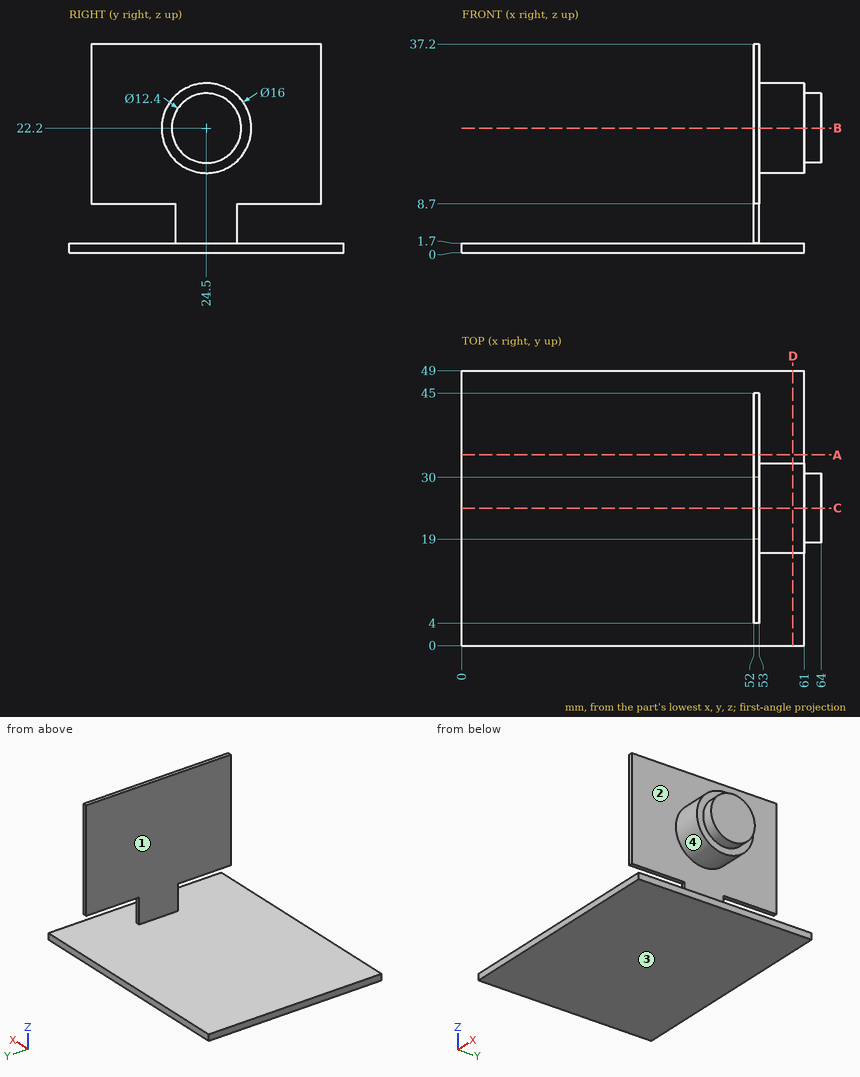
The drawing under review shows one solid part. Ordinate dimensions are in mm from its lowest x, y, z. Coordinates: 2 decimals unless noted, no trailing zeros. Write each loop counter-clockwise with the first axis right and the second up, starting at its lowest first coordinate (ties: lowest second). Pieces come first, ordered by that corner, then holes.
1) Mouldability with a two-part tool opening along Z and no side actions: class the marked faces 1, 2, 3 and 4 as +Z half, -Z half, draft (parallel to the pull), parting line (faces both ways), or undercut.
2) Add section B-B (z = 22.2). Write out the cut boundary in (x, y), plus the area to 3 significant figures.
3) To check wall thickness, follow L1, parallel to Z at x = 39, y = 41.5; L2, parallel to X at y = 23.5, z = 10.5; L3, parallel to X at y = 28, z = 17. State the ranges of each line that lie inside material, in increasing order.
4) Add section C-C (y = 24.5). Write out the cut boundary in (x, z), plus the area to 3 significant figures.
5) Add section D-D (x = 59). Write out the cut boundary in (y, z), plus the area to 3 significant figures.
6) Insertion check: pin 1 (1.9 mm diameter, centred on y = 25.5, z = 0.5, fed in from +X); pin 2 (6 mm diameter, centred on y = 5.5, z = 33.5, fed in from -X); pin 3 (24.5 mm diameter, centred on x = 25, y = 16.5, fed in from +Z). Each pin has a flat end and moves straight along its axis. Give the tip position at first contact, or say it passes through.
7) Add section A-A (y = 34). Write out the cut boundary in (x, z), plus the area to 3 significant figures.
Check result:
1. face 1: draft
1. face 2: undercut
1. face 3: -Z half
1. face 4: undercut
2. outline: (52, 4) - (53, 4) - (53, 16.5) - (61, 16.5) - (61, 18.3) - (64, 18.3) - (64, 30.7) - (61, 30.7) - (61, 32.5) - (53, 32.5) - (53, 45) - (52, 45) - close
2. area: 206 mm2
3. L1: z = 0 to 1.7
3. L2: x = 52 to 53
3. L3: x = 52 to 61
4. outline: (0, 0) - (61, 0) - (61, 1.7) - (53, 1.7) - (53, 14.2) - (61, 14.2) - (61, 16) - (64, 16) - (64, 28.4) - (61, 28.4) - (61, 30.2) - (53, 30.2) - (53, 37.2) - (52, 37.2) - (52, 1.7) - (0, 1.7) - close
4. area: 304 mm2
5. outline: (0, 0) - (49, 0) - (49, 1.7) - (0, 1.7) - close; circle Ø16 at (24.5, 22.2)
5. area: 284 mm2
6. pin 1: stops at x = 61
6. pin 2: stops at x = 52
6. pin 3: stops at z = 1.7
7. outline: (0, 0) - (61, 0) - (61, 1.7) - (0, 1.7) - close; (52, 8.7) - (53, 8.7) - (53, 37.2) - (52, 37.2) - close
7. area: 132 mm2
